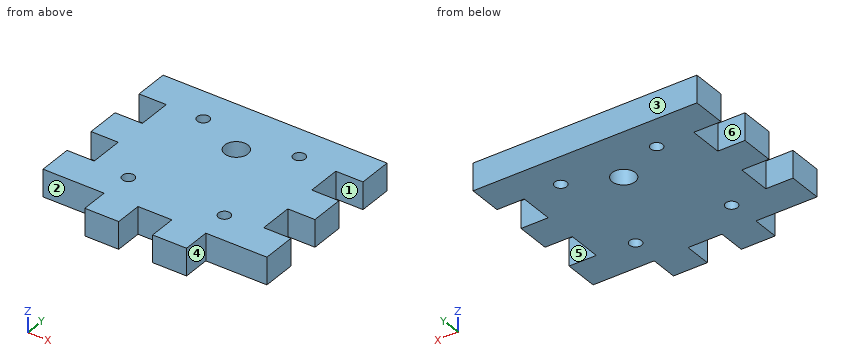
```python
from build123d import *

# Parameters (mm, degrees)
SKETCH1_R           = 1.397
SKETCH1_R_2         = 2.704093878
BOSS_EXTRUDE1_DEPTH = 6.35


with BuildPart() as part:
    # Sketch1 → Boss-Extrude1 (new body)
    with BuildSketch(Plane.XY):
        Polygon((34.222577161, -16.34309441), (34.222577161, -24.260672631), (40.572577161, -24.260672631), (40.572577161, -32.178250852), (34.222577161, -32.178250852), (26.30499894, -32.178250852), (26.30499894, -38.528250852), (18.387420719, -38.528250852), (18.387420719, -32.178250852), (10.469842498, -32.178250852), (10.469842498, -38.528250852), (2.552264276, -38.528250852), (2.552264276, -32.178250852), (-5.365313945, -32.178250852), (-11.715313945, -32.178250852), (-11.715313945, -24.260672631), (-5.365313945, -24.260672631), (-5.365313945, -16.34309441), (-11.715313945, -16.34309441), (-11.715313945, -8.425516188), (-5.365313945, -8.425516188), (-5.365313945, -0.507937967), (-11.715313945, -0.507937967), (-11.715313945, 7.409640254), (40.572577161, 7.409640254), (40.572577161, -0.507937967), (34.222577161, -0.507937967), (34.222577161, -8.425516188), (40.572577161, -8.425516188), (40.572577161, -16.34309441), align=None)
        with Locations((3.220865479, -0.422913296)):
            Circle(SKETCH1_R, mode=Mode.SUBTRACT)
        with Locations((25.636397737, -0.422913296)):
            Circle(SKETCH1_R, mode=Mode.SUBTRACT)
        with Locations((25.636397737, -25.106684096)):
            Circle(SKETCH1_R, mode=Mode.SUBTRACT)
        with Locations((3.220865479, -25.106684096)):
            Circle(SKETCH1_R, mode=Mode.SUBTRACT)
        with Locations((14.428631608, -5.359667456)):
            Circle(SKETCH1_R_2, mode=Mode.SUBTRACT)
    extrude(amount=BOSS_EXTRUDE1_DEPTH)


solid = part.part
```
Work out the finished part from the listing and answer in its coordinate system (mm). Face numbers are marked on the shaded views. A direction names the side the tool comes from. Round coordinates to 2 decimals unless told otherwise and drop trailing zeros. Write each loop counter-clockwise with the first axis right and the second up, starting at its lowest first coordinate (ties: lowest second). Pieces come first, ordered by that corner, then holes. Notation, with made-up numbers: (53.25, 80) -> (94.25, 80) arc R17 ccw to (94.25, 90) -> close; hole circle Ø6 at (88.25, 24). An arc over 180 degrees is marked (long way). Write each question's results on one line, items separated by ' | '.
Q1. Determine the mould class of the marked faces 1, 2 and 3 for opening direction Y: released by +Y, released by -Y, zero draft, split by the parting line, or undercut.
Data:
face 1: undercut | face 2: released by -Y | face 3: released by +Y
Q2. Section B-B, the plane z = 2.5 is taken. Give the number of separate pieces and of enclosed holes in the cut face, then the cut area to 3 significant figures.
Data:
separate pieces: 1 | enclosed holes: 5 | area: 1,920 mm^2
Q3. Which of the six approach directions +Z, -Z, +X, -X, +Y, -Y give full straight-line access (tool end or side, diameter ignored) to the marked faces 4, 5 and 6?
Data:
face 4: +Z, -Z, +X, -Y | face 5: +Z, -Z, +X | face 6: +Z, -Z, -X
Q4. Flat-ended cylindrical pins translate along their axes: P1, Ø1.9, axis at y = -21, z = 4, coming from the -X side; P2, Ø1.9, axis at y = -3.5, z = 3, coming from the +X side; P3, Ø3, axis at x = 38.5, z = 3, coming from the -Y side. Find the tip coordinate at first contact, or state that the pin passes through.
Data:
P1: x = -5.37 | P2: x = 34.22 | P3: y = -32.18
Q5. Straight lines are drawn through the part: line 1 along Y through (x, z) = (37, 3.25); line 2 along X through (y, z) = (-25, 2.75); line 3 along Y through (x, z) = (4.5, 0.75). For each, find the intervals that lie inside material, in ascending order. Write a range as [from, to].
Data:
line 1: [-32.18, -24.26], [-16.34, -8.43], [-0.51, 7.41] | line 2: [-11.72, 1.83], [4.61, 24.24], [27.03, 40.57] | line 3: [-38.53, -25.67], [-24.55, -0.98], [0.14, 7.41]
Q6. Section C-C, the plane y = -22 is taken. Write down the section's boundary in (x, z).
Data:
outline: (-5.37, 0) -> (34.22, 0) -> (34.22, 6.35) -> (-5.37, 6.35) -> close
Q7. Section D-D, the plane x = -2 is taken. Write down the section's boundary in (y, z).
Data:
outline: (-32.18, 0) -> (7.41, 0) -> (7.41, 6.35) -> (-32.18, 6.35) -> close
Q8. Section A-A, the plane x = 37 is taken. Write down the section's boundary in (y, z).
Data:
outline: (-32.18, 0) -> (-24.26, 0) -> (-24.26, 6.35) -> (-32.18, 6.35) -> close; (-16.34, 0) -> (-8.43, 0) -> (-8.43, 6.35) -> (-16.34, 6.35) -> close; (-0.51, 0) -> (7.41, 0) -> (7.41, 6.35) -> (-0.51, 6.35) -> close
